For this review, take the finished solid that the model builds, in its own axes (mm). A direction names the side the tool comes from. Coordinates: 2 decimals unless noted, no trailing zeros. Loops run counter-clockwise (first coordinate to the right, second up) from the corner with the lowest first, then second, coordinate; pieces in that order, holes last. Notation, with made-up numbers: M 32,10 L 72,10 A22 ccw 72,33 Z; hole C 3,25.5 d9. An arc over 180 degrees is marked long. Answer as a JSON object with one key per item and string values. Group by question number.
Item 1: Add section C-C (x = 2.5). State the section outline as (y, z) points, then the cut area to 3 significant figures.
Item 2: Mouldability with a two-part tool opening along Y and no side actions: class faces 1 (the face through (5, 47, -20)), 2 (the face through (10.106, 44.285, -18.699)), 3 (the face through (20.5, 30, -1)) as +Y half, -Y half, draft (parallel to the pull), parting line (faces both ways), or undercut.
Item 3: Wall thickness on L1, parallel to Y at x = 13, z = -7; L2, parallel to Z at x = 3.5, y = 15.5; L3, parallel to Y at x = 15.5, z = -19.8: over which ranges is each line inside the solid? List them lowest first. Write a range as from..to.
Item 4: Add section B-B (x = 15.5). State the section outline as (y, z) points.
Item 5: Add section A-A (y = 48.5). State the section outline as (x, z) points, then the cut area to 3 significant figures.
Item 6: Tool access review of faces 4 (the face through (10, 48, -19)), 5 (the face through (10, 21, 0)), 6 (the face through (10, 42, -11)): name each direction out of +Z, -Z, +X, -X, +Y, -Y from which nothing blocks a thin tool from reaching the whole face with its end or side.
Item 7: Add section D-D (z = -12.25). State the section outline as (x, y) points, then the cut area to 3 significant figures.
Item 8: Insertion check: pin 1 (2.5 mm diameter, centred on x = 15.5, y = 48.5, fed in from +Z); pin 2 (1.5 mm diameter, centred on x = 17, z = -5.5, fed in from -Y); pin 3 (4 mm diameter, centred on x = 5, y = 48.5, fed in from +Z); pin 4 (4 mm diameter, centred on x = 6.5, y = 8, fed in from -Z). Each pin has a flat end and moves straight along its axis. Give the tip position at first contact, or say it passes through.
from build123d import *

# Parameters (mm, degrees)
BOSS_EXTRUDE1_DEPTH = 20.5
SKETCH2_R           = 1.5
CUT_EXTRUDE1_DEPTH  = 60.036005962


with BuildPart() as part:
    # Sketch1 → Boss-Extrude1 (new body)
    with BuildSketch(Plane(origin=(0, 0, 0), x_dir=(0, 0, -1), z_dir=(1, 0, 0))):
        with BuildLine():
            Line((0, 0), (0, 43))
            ThreePointArc((0, 43), (0.292893219, 43.707106781), (1, 44))
            Line((1, 44), (18, 44))
            ThreePointArc((18, 44), (18.707106781, 44.292893219), (19, 45))
            Line((19, 45), (19, 52))
            Line((19, 52), (21, 52))
            Line((21, 52), (21, 44))
            ThreePointArc((21, 44), (20.414213562, 42.585786438), (19, 42))
            Line((19, 42), (2, 42))
            Line((2, 42), (2, 0))
            Line((2, 0), (0, 0))
        make_face()
    extrude(amount=BOSS_EXTRUDE1_DEPTH)

    # Sketch2 → Cut-Extrude1 (cut, through all)
    with BuildSketch(Plane.XY.offset(-19)):
        with Locations((5, 48.5)):
            Circle(SKETCH2_R)
        with Locations(Location((15.5, 48.5, 0), (0, 0, 180))):
            Circle(SKETCH2_R)
    extrude(amount=-CUT_EXTRUDE1_DEPTH, mode=Mode.SUBTRACT)


solid = part.part
From the geometry:
{
 "1": {"outline": "M 0,-2 L 42,-2 L 42,-19 A2 ccw 44,-21 L 52,-21 L 52,-19 L 45,-19 A1 cw 44,-18 L 44,-1 A1 ccw 43,0 L 0,0 Z", "area": "141 mm²"},
 "2": {"face 1": "undercut", "face 2": "+Y half", "face 3": "draft"},
 "3": {"L1": "y = 42..44", "L2": "z = -2..0", "L3": "y = 42.17..47, 50..52"},
 "4": {"outline": "M 0,-2 L 42,-2 L 42,-19 A2 ccw 44,-21 L 47,-21 L 47,-19 L 45,-19 A1 cw 44,-18 L 44,-1 A1 ccw 43,0 L 0,0 Z; M 50,-21 L 52,-21 L 52,-19 L 50,-19 Z"},
 "5": {"outline": "M 0,-21 L 3.5,-21 L 3.5,-19 L 0,-19 Z; M 6.5,-21 L 14,-21 L 14,-19 L 6.5,-19 Z; M 17,-21 L 20.5,-21 L 20.5,-19 L 17,-19 Z", "area": "29.0 mm²"},
 "6": {"face 4": "+Z, +X, -X, +Y", "face 5": "+Z, +X, -X, +Y, -Y", "face 6": "-Z, +X, -X, -Y"},
 "7": {"outline": "M 0,42 L 20.5,42 L 20.5,44 L 0,44 Z", "area": "41.0 mm²"},
 "8": {"pin 1": "passes through", "pin 2": "stops at y = 42", "pin 3": "stops at z = -19", "pin 4": "stops at z = -2"}
}
